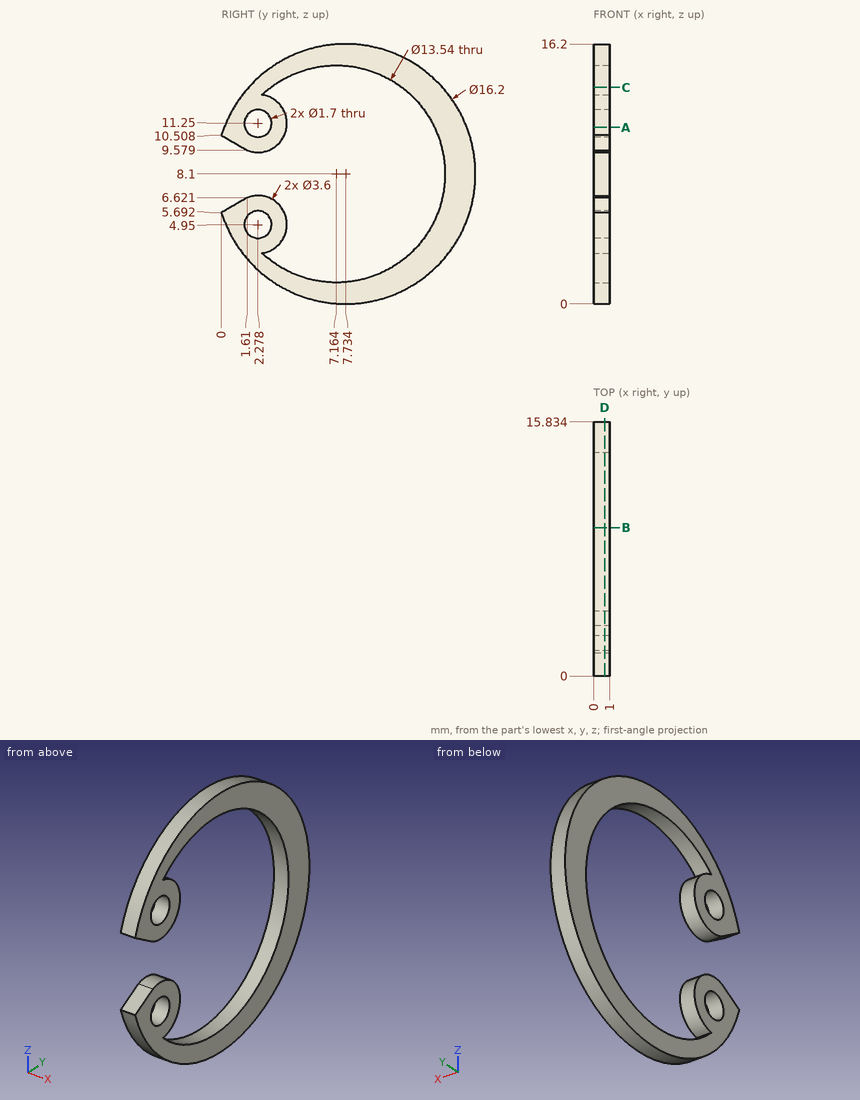
Can you work these out from the drawing? Everything is in mm from the part's minimum corner. Round coordinates to 2 decimals unless told otherwise and drop trailing zeros. Loops run counter-clockwise (first coordinate to the right, second up) from the corner with the lowest first, then second, coordinate; pieces in that order, holes last. Notation, with made-up numbers: (31.5, -2.5) -> (36.5, -2.5) arc R25 cw to (36.5, 31.5) -> close; hole circle Ø9 at (84.5, 80.25). An arc over 180 degrees is marked (long way). Answer in a Markdown table with one row per item.
Item 1: Suppose I cut it at A-A, the plane z = 11. List the corners of the cut face in (x, y) for me (1 decimal).
Answer block:
| item | result |
|---|---|
| outline | (0, 0.2) -> (1, 0.2) -> (1, 1.5) -> (0, 1.5) -> close; (0, 3.1) -> (1, 3.1) -> (1, 4.1) -> (0, 4.1) -> close; (0, 13.3) -> (1, 13.3) -> (1, 15.3) -> (0, 15.3) -> close |
Item 2: Suppose I cut it at B-B, the plane y = 9.25. List the corners of the cut face in (x, z) for me.
Answer block:
| item | result |
|---|---|
| outline | (0, 0.14) -> (1, 0.14) -> (1, 1.66) -> (0, 1.66) -> close; (0, 14.54) -> (1, 14.54) -> (1, 16.06) -> (0, 16.06) -> close |
Item 3: Suppose I cut it at D-D, the plane x = 0.7. List the corners of the cut face in (y, z) for me.
Answer block:
| item | result |
|---|---|
| outline | (0, 5.69) arc R8.1 ccw (long way) to (0, 10.51) -> (1.61, 9.58) arc R1.8 ccw (long way) to (2.53, 13.03) arc R6.77 cw (long way) to (2.53, 3.17) arc R1.8 ccw (long way) to (1.61, 6.62) -> close; hole circle Ø1.7 at (2.28, 4.95); hole circle Ø1.7 at (2.28, 11.25) |
Item 4: If I drill on probe 1 along Z at (x, y) = (0.7, 3.25) (1 decimal); probe 2 along Y at (x, z) = (0.5, 11.25) (1 decimal); probe 3 along Y at (x, z) = (0.5, 12) (1 decimal), over which ranges is the centre line in solid material (lowest first)?
Answer block:
| item | result |
|---|---|
| probe 1 | 1.4 to 2.6, 3.4 to 6.5, 9.7 to 12.8, 13.6 to 14.8 |
| probe 2 | 0.3 to 1.4, 3.1 to 4.1, 13.2 to 15.2 |
| probe 3 | 0.6 to 1.9, 2.7 to 3.9, 12.7 to 14.8 |
Item 5: Suppose I cut it at C-C, the plane z = 13.5. List the corners of the cut face in (x, y) for me.
Answer block:
| item | result |
|---|---|
| outline | (0, 1.7) -> (1, 1.7) -> (1, 3.08) -> (0, 3.08) -> close; (0, 11.25) -> (1, 11.25) -> (1, 13.77) -> (0, 13.77) -> close |
